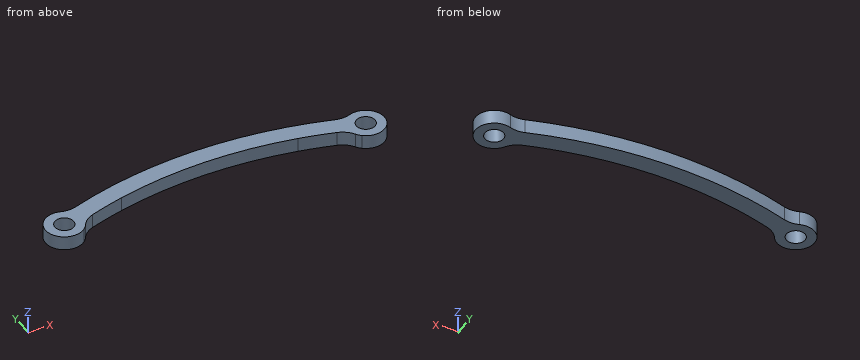
```python
from build123d import *

# Parameters (mm, degrees)
SKETCH_1_R          = 8
EXTRUDE_1_DEPTH     = 6
SKETCH_2_R          = 4
CUT_EXTRUDE_1_DEPTH = 15
FILLET_1_R          = 10
EXTRUDE_START       = -6
EXTRUDE_3_DEPTH     = 6
CUT_EXTRUDE_START   = -6
CUT_EXTRUDE_2_DEPTH = 6
FILLET_2_R          = 10


with BuildPart() as part:
    # 草图1 → 凸台-拉伸1 (new body)
    with BuildSketch(Plane.XY):
        with Locations((-65, 0)):
            Circle(SKETCH_1_R)
        with Locations((65, 0)):
            Circle(SKETCH_1_R)
        with BuildLine():
            Line((-65, 4), (65, 4))
            ThreePointArc((65, 4), (69, 0), (65, -4))
            Line((65, -4), (-65, -4))
            ThreePointArc((-65, -4), (-69, 0), (-65, 4))
        make_face()
    extrude(amount=EXTRUDE_1_DEPTH)

    # 草图2 → 切除-拉伸1 (cut)
    with BuildSketch(Plane.XY.offset(6)):
        with Locations((-65, 0)):
            Circle(SKETCH_2_R)
        with Locations((65, 0)):
            Circle(SKETCH_2_R)
    extrude(amount=-CUT_EXTRUDE_1_DEPTH, mode=Mode.SUBTRACT)

    # 圆角1
    fillet_1_edges = [part.edges().sort_by_distance(p)[0] for p in [
        (58.07179677, -4, 3),
        (-58.07179677, -4, 3),
        (-58.07179677, 4, 3),
        (58.07179677, 4, 3),
    ]]
    fillet(fillet_1_edges, radius=FILLET_1_R)

    # 草图4 → 凸台-拉伸3 (add)
    with BuildSketch(Plane.XY.offset(6).offset(EXTRUDE_START)):
        with BuildLine():
            ThreePointArc((53.536596581, 4), (0, 12.145896684), (-53.536596581, 4))
            Line((-53.536596581, 4), (-37.975876204, 4))
            ThreePointArc((-37.975876204, 4), (0, 8.145896684), (37.975876204, 4))
            Line((37.975876204, 4), (53.536596581, 4))
        make_face()
        with BuildLine():
            ThreePointArc((59.862982118, 6.135618714), (0, 16.145896684), (-59.862982118, 6.135618714))
            ThreePointArc((-59.862982118, 6.135618714), (-56.954026736, 4.54897326), (-53.686291501, 4))
            Line((-53.686291501, 4), (-53.536596581, 4))
            ThreePointArc((-53.536596581, 4), (0, 12.145896684), (53.536596581, 4))
            Line((53.536596581, 4), (53.686291501, 4))
            ThreePointArc((53.686291501, 4), (56.954026736, 4.54897326), (59.862982118, 6.135618714))
        make_face()
    extrude(amount=EXTRUDE_3_DEPTH)

    # 草图5 → 切除-拉伸2 (cut)
    with BuildSketch(Plane.XY.offset(6).offset(CUT_EXTRUDE_START)):
        with BuildLine():
            ThreePointArc((-59.971685112, -6.222222222), (-57.019624834, -4.571909584), (-53.686291501, -4))
            Line((-53.686291501, -4), (53.686291501, -4))
            ThreePointArc((53.686291501, -4), (57.019624834, -4.571909584), (59.971685112, -6.222222222))
            ThreePointArc((59.971685112, -6.222222222), (58.106897, -4.060188546), (57.120098961, -1.380999498))
            ThreePointArc((57.120098961, -1.380999498), (47.624047624, 1.580102463), (37.975876204, 4))
            Line((37.975876204, 4), (-37.975876204, 4))
            ThreePointArc((-37.975876204, 4), (-47.624047624, 1.580102463), (-57.120098961, -1.380999498))
            ThreePointArc((-57.120098961, -1.380999498), (-58.106897, -4.060188546), (-59.971685112, -6.222222222))
        make_face()
    extrude(amount=CUT_EXTRUDE_2_DEPTH, mode=Mode.SUBTRACT)

    # 圆角2
    fillet_2_edges = [part.edges().sort_by_distance(p)[0] for p in [
        (-57.120098961, -1.380999498, 3),
    ]]
    fillet(fillet_2_edges, radius=FILLET_2_R)
    fillet_2_2_edges = [part.edges().sort_by_distance(p)[0] for p in [
        (59.862982118, 6.135618714, 3),
    ]]
    fillet(fillet_2_2_edges, radius=FILLET_2_R)
    fillet_2_3_edges = [part.edges().sort_by_distance(p)[0] for p in [
        (57.120098961, -1.380999498, 3),
    ]]
    fillet(fillet_2_3_edges, radius=FILLET_2_R)
    fillet_2_4_edges = [part.edges().sort_by_distance(p)[0] for p in [
        (-59.862982118, 6.135618714, 3),
    ]]
    fillet(fillet_2_4_edges, radius=FILLET_2_R)


solid = part.part
```
The listing builds one solid part. Answer for the finished solid, in the listing's coordinates (mm). Coordinates: 2 decimals unless noted, no trailing zeros. Write each loop counter-clockwise with the first axis right and the second up, starting at its lowest first coordinate (ties: lowest second). Pieces come first, ordered by that corner, then holes. Notation, with made-up numbers: M 26,-31 L 40,-31 A7 ccw 40,-19 Z; hole C 36.25,-26 d8. An arc over 180 degrees is marked long. Use a Markdown table: item, result. Add a question column.
1. Section D-D (x = 50) is taken. Give the vertices of the cut face in (y, z), plus the area to 3 significant figures.
2. Given P1, Ø6.5, axis at x = 65, y = 0, coming from the -Z side; P2, Ø3, axis at x = 32, z = 2.5, coming from the -Y side; P3, Ø3, axis at x = -51.5, z = 4.5, coming from the -Y side; P4, Ø1.5, axis at x = -29, z = 4, coming from the +Y side, each flat-ended and moving along its own axis, determine where each tip first touches the part or whether it passes through.
3. Section C-C (y = 11) is taken. Give the vertices of the cut face in (x, z), plus the area to 3 significant figures.
4. Straight lines are drawn through the part: line 1 along X through (y, z) = (-3.5, 5.75); line 2 along Y through (x, z) = (-65, 2.85); line 3 along X through (y, z) = (-4.75, 2.25). For each, find the intervals that lie inside material, in ascending order. Write a range as [from, to].
5. Section A-A (x = -65) is taken. Give the vertices of the cut face in (y, z), plus the area to 3 significant figures.
6. Section B-B (z = 2.25) is taken. Count the separate pieces of the cut face and the enclosed holes in it, plus the area to 3 significant figures.
Data:
| question | item | result |
|---|---|---|
| 1 | outline | M 0.89,0 L 9.22,0 L 9.22,6 L 0.89,6 Z |
| 1 | area | 50.0 mm2 |
| 2 | P1 | passes through |
| 2 | P2 | stops at y = 4.93 |
| 2 | P3 | stops at y = -0.03 |
| 2 | P4 | stops at y = 13.96 |
| 3 | outline | M -43.21,0 L 43.21,0 L 43.21,6 L -43.21,6 Z |
| 3 | area | 519 mm2 |
| 4 | line 1 | x = [-72.19, -66.94], [-63.06, -57.72], [57.72, 63.06], [66.94, 72.19] |
| 4 | line 2 | y = [-8, -4], [4, 8] |
| 4 | line 3 | x = [-71.44, -58.56], [58.56, 71.44] |
| 5 | outline | M -8,0 L -4,0 L -4,6 L -8,6 Z; M 4,0 L 8,0 L 8,6 L 4,6 Z |
| 5 | area | 48.0 mm2 |
| 6 | separate pieces | 1 |
| 6 | enclosed holes | 2 |
| 6 | area | 1,250 mm2 |
